Geometry: final body of the model. Coordinates: model frame, mm. Face numbers are marked on the shaded views. Give positions to 0.01 mm unless a question says otherwise; leave off trailing zeros. Order: outer loops, then holes, each group sorted by start corner. A loop starts at its lowest first (then second) coordinate and runs counter-clockwise, first axis right, second up. Notation, with made-up numbers: (37.5, 72.25) -> (90.5, 72.25) arc R15 cw to (90.5, 90.25) -> close; hole circle Ø10 at (-39.75, 62.25). An arc over 180 degrees is marked (long way). Write item = value, one per line.
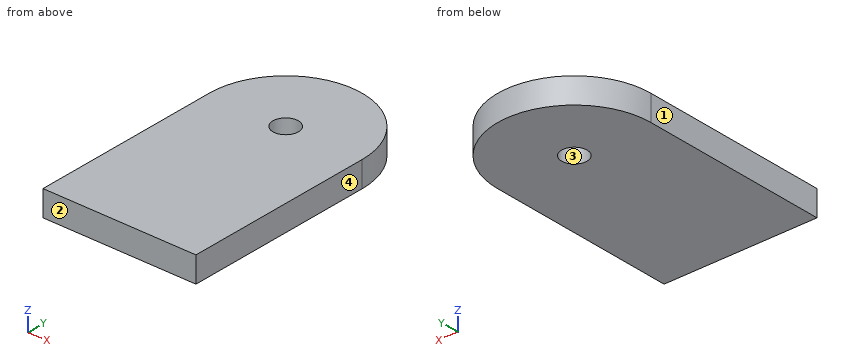
```python
from build123d import *

# Parameters (mm, degrees)
CROQUIS1_R              = 5
SALIENTE_EXTRUIR1_DEPTH = 10


with BuildPart() as part:
    # Croquis1 → Saliente-Extruir1 (new body)
    with BuildSketch(Plane.XY):
        with BuildLine():
            Line((9.5, -75), (-30, -75))
            Line((-30, -75), (-30, 0))
            ThreePointArc((-30, 0), (0, 30), (30, 0))
            Line((30, 0), (30, -75))
            Line((30, -75), (9.5, -75))
        make_face()
        Circle(CROQUIS1_R, mode=Mode.SUBTRACT)
    extrude(amount=SALIENTE_EXTRUIR1_DEPTH)


solid = part.part
```
1) Line query: line 1 (Y direction, x = 0, z = 5); line 2 (X direction, y = 3.5, z = 7.5); line 3 (Y direction, x = 19, z = 0.75). Output: solid intervals per line, ascending. Write a range as from..to.
Check sheet entries:
line_1 = -75..-5, 5..30
line_2 = -29.8..-3.57, 3.57..29.8
line_3 = -75..23.22
2) Section query B-B (z = 2.25). Output: boundary loops of the cut face in (x, y).
Check sheet entries:
outline = (-30, -75) -> (30, -75) -> (30, 0) arc R30 ccw to (-30, 0) -> close; hole circle Ø10 at (0, 0)
3) Section query D-D (y = 21). Output: boundary loops of the cut face in (x, z).
Check sheet entries:
outline = (-21.42, 0) -> (21.42, 0) -> (21.42, 10) -> (-21.42, 10) -> close
4) First-contact query: P1, Ø6, axis at x = 14.5, z = 7, coming from the +Y side. Flat tip, straight axial feed; report the tip coordinate or a pass-through.
Check sheet entries:
P1 = 27.71
5) Mould query, pull axis X, two halves, no side actions, for the marked faces 1, 2, 3 and 4. Classes: +X half, -X half, draft (parallel to the pull), parting line (faces both ways), or undercut.
Check sheet entries:
face_1 = -X half
face_2 = draft
face_3 = undercut
face_4 = +X half
6) Section query A-A (x = 0). Output: boundary loops of the cut face in (y, z), plus the area to 3 significant figures.
Check sheet entries:
outline = (-75, 0) -> (-5, 0) -> (-5, 10) -> (-75, 10) -> close; (5, 0) -> (30, 0) -> (30, 10) -> (5, 10) -> close
area = 950 mm²
7) Section query C-C (y = 2). Output: boundary loops of the cut face in (x, z), plus the area to 3 significant figures.
Check sheet entries:
outline = (-29.93, 0) -> (-4.58, 0) -> (-4.58, 10) -> (-29.93, 10) -> close; (4.58, 0) -> (29.93, 0) -> (29.93, 10) -> (4.58, 10) -> close
area = 507 mm²
